Can you work these out from the model? Positions are in its coordinate system, mm. Face numbers are marked on the shaded views. A direction names the side the tool comes from. Round coordinates to 2 decimals unless told otherwise and drop trailing zeros. Write each loop counter-clockwise with the first axis right and the second up, starting at its lowest first coordinate (ties: lowest second). Pieces come first, ordered by that corner, then holes.
Q1. If we section it at C-C (y = 19.5): Please give me the cut outline in (x, z).
Q2. If we section it at B-B (z = 6.25): Please give me the cut outline in (x, y), plus the area to 3 significant figures.
Q3. If we section it at A-A (x = 0): Please give me the cut outline in (y, z), plus the area to 3 significant figures.
Q4. I'm going to push flat-ended pins straight in: pin 1 Ø2 at (y, z) = (-9.5, 16.5) entering from +X; pin 2 Ø12 at (x, z) = (12.5, 4.5) entering from -Y; pin 3 Ø6 at (y, z) = (5, 5) entering from +X. Where does each tip first touch, or does it pass through?
Q5. Please list where these lines run through material, in increasing order: line 1 along X through (y, z) = (-0.5, 9); line 2 along Y through (x, z) = (-22.5, 2.5); line 3 along Z through (x, y) = (16.5, -20).
Q6. For the marked faces 1, 2, 3, 4 and 5, which set-ups out of +Z, -Z, +X, -X, +Y, -Y let a thin tool reach every point of the face, with its end or its side?
Q7. If we section it at D-D (x = 21): Please give me the cut outline in (y, z).
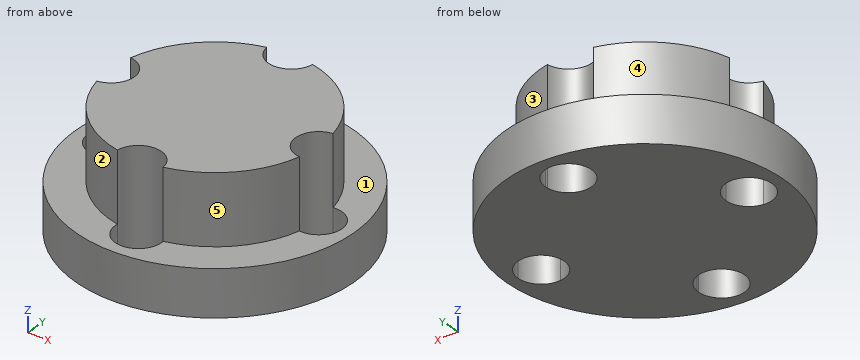
from build123d import *

# Parameters (mm, degrees)
F1_DEPTH = 25
F0_R     = 30
F2_DEPTH = 10


with BuildPart() as f1:
    # F0 (on Top) → F1 (new body)
    with BuildSketch(Plane.XY):
        with BuildLine():
            ThreePointArc((21.9444444444, -4.96903995), (17.5, 0), (21.9444444444, 4.96903995))
            ThreePointArc((21.9444444444, 4.96903995), (15.9099025767, 15.9099025767), (4.96903995, 21.9444444444))
            ThreePointArc((4.96903995, 21.9444444444), (0, 17.5), (-4.96903995, 21.9444444444))
            ThreePointArc((-4.96903995, 21.9444444444), (-15.9099025767, 15.9099025767), (-21.9444444444, 4.96903995))
            ThreePointArc((-21.9444444444, 4.96903995), (-18.7732200375, 3.3333333333), (-17.5, 0))
            ThreePointArc((-17.5, 0), (-18.7732200375, -3.3333333333), (-21.9444444444, -4.96903995))
            ThreePointArc((-21.9444444444, -4.96903995), (-15.9099025767, -15.9099025767), (-4.96903995, -21.9444444444))
            ThreePointArc((-4.96903995, -21.9444444444), (0, -17.5), (4.96903995, -21.9444444444))
            ThreePointArc((4.96903995, -21.9444444444), (15.9099025767, -15.9099025767), (21.9444444444, -4.96903995))
        make_face()
    extrude(amount=F1_DEPTH)

    # F0 (on Top) → F2 (join)
    with BuildSketch(Plane.XY):
        Circle(F0_R)
        with BuildLine():
            ThreePointArc((4.96903995, 21.9444444444), (15.9099025767, 15.9099025767), (21.9444444444, 4.96903995))
            ThreePointArc((21.9444444444, 4.96903995), (25.8333333333, 3.7267799625), (27.5, 0))
            ThreePointArc((27.5, 0), (25.8333333333, -3.7267799625), (21.9444444444, -4.96903995))
            ThreePointArc((21.9444444444, -4.96903995), (15.9099025767, -15.9099025767), (4.96903995, -21.9444444444))
            ThreePointArc((4.96903995, -21.9444444444), (4.9922539874, -22.2217912205), (5, -22.5))
            ThreePointArc((5, -22.5), (-0.2782087795, -27.4922539874), (-4.96903995, -21.9444444444))
            ThreePointArc((-4.96903995, -21.9444444444), (-15.9099025767, -15.9099025767), (-21.9444444444, -4.96903995))
            ThreePointArc((-21.9444444444, -4.96903995), (-27.5, 0), (-21.9444444444, 4.96903995))
            ThreePointArc((-21.9444444444, 4.96903995), (-15.9099025767, 15.9099025767), (-4.96903995, 21.9444444444))
            ThreePointArc((-4.96903995, 21.9444444444), (-0.2782087795, 27.4922539874), (5, 22.5))
            ThreePointArc((5, 22.5), (4.9922539874, 22.2217912205), (4.96903995, 21.9444444444))
        make_face(mode=Mode.SUBTRACT)
    extrude(amount=F2_DEPTH)


solid = f1.part
A:
1. outline: (-22.8, 0) - (-4, 0) - (-4, 25) - (-11.22, 25) - (-11.22, 10) - (-22.8, 10) - close; (4, 0) - (22.8, 0) - (22.8, 10) - (11.22, 10) - (11.22, 25) - (4, 25) - close
2. outline: circle Ø60 at (0, 0); hole circle Ø10 at (-22.5, 0); hole circle Ø10 at (0, -22.5); hole circle Ø10 at (0, 22.5); hole circle Ø10 at (22.5, 0)
2. area: 2,510 mm2
3. outline: (-30, 0) - (-27.5, 0) - (-27.5, 10) - (-30, 10) - close; (-17.5, 0) - (17.5, 0) - (17.5, 25) - (-17.5, 25) - close; (27.5, 0) - (30, 0) - (30, 10) - (27.5, 10) - close
3. area: 925 mm2
4. pin 1: stops at x = 20.83
4. pin 2: stops at y = -29.29
4. pin 3: stops at x = 29.93
5. line 1: x = -30 to -27.47, -17.53 to 17.53, 27.47 to 30
5. line 2: y = -19.84 to -5, 5 to 19.84
5. line 3: z = 0 to 10
6. face 1: +Z
6. face 2: +Z, -X, -Y
6. face 3: +Z, +X, +Y
6. face 4: +Z, -X, +Y
6. face 5: +Z, +X, -Y
7. outline: (-21.42, 0) - (-4.77, 0) - (-4.77, 25) - (-8.08, 25) - (-8.08, 10) - (-21.42, 10) - close; (4.77, 0) - (21.42, 0) - (21.42, 10) - (8.08, 10) - (8.08, 25) - (4.77, 25) - close
